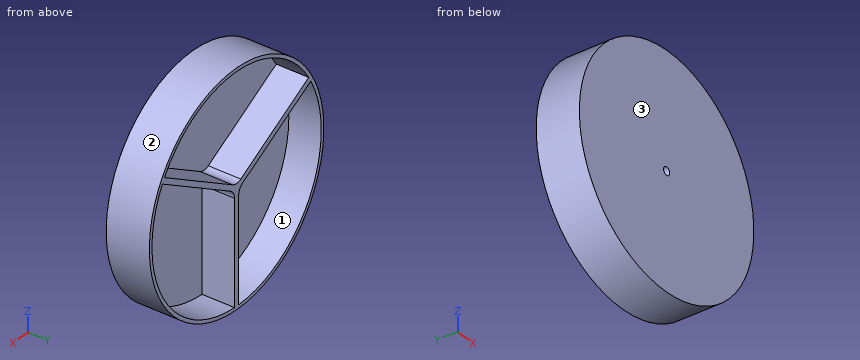
```python
from build123d import *

# Parameters (mm, degrees)
BOSS_EXTRUDE2_DEPTH   = 8
BOSS_EXTRUDE2_2_DEPTH = 8
BOSS_EXTRUDE2_3_DEPTH = 8
SKETCH2_4_R           = 84
BOSS_EXTRUDE3_DEPTH   = 32
SKETCH4_R             = 2.95
CUT_EXTRUDE2_DEPTH    = 8


with BuildPart() as part:
    # Sketch2 → Boss-Extrude2 (new body)
    with BuildSketch(Plane(origin=(0, 0, 0), x_dir=(1, 0, 0), z_dir=(0, 1, 0))):
        with BuildLine():
            Line((-2, 5.579606434), (-2, 81.475456427))
            ThreePointArc((-2, 81.475456427), (-70.623024312, 40.677247166), (-71.479275287, -39.15307401))
            Line((-71.479275287, -39.15307401), (-6, -1.348596796))
            ThreePointArc((-6, -1.348596796), (-3.07179677, 1.579606434), (-2, 5.579606434))
        make_face()
    extrude(amount=BOSS_EXTRUDE2_DEPTH)



with BuildPart() as body_2:
    # Sketch2 → Boss-Extrude2 2 (new body)
    with BuildSketch(Plane(origin=(0, 0, 0), x_dir=(1, 0, 0), z_dir=(0, 1, 0))):
        with BuildLine():
            ThreePointArc((81.5, 0), (58.332023795, 56.917703748), (2, 81.475456427))
            Line((2, 81.475456427), (2, 5.579606434))
            ThreePointArc((2, 5.579606434), (3.07179677, 1.579606434), (6, -1.348596796))
            Line((6, -1.348596796), (71.479275287, -39.15307401))
            ThreePointArc((71.479275287, -39.15307401), (78.95508513, -20.207536516), (81.5, 0))
        make_face()
    extrude(amount=BOSS_EXTRUDE2_2_DEPTH)


with BuildPart() as body_3:
    # Sketch2 → Boss-Extrude2 3 (new body)
    with BuildSketch(Plane(origin=(0, 0, 0), x_dir=(1, 0, 0), z_dir=(0, 1, 0))):
        with BuildLine():
            Line((-4, -4.812698411), (-69.472135836, -42.613053661))
            ThreePointArc((-69.472135836, -42.613053661), (0, -81.5), (69.472135836, -42.613053661))
            Line((69.472135836, -42.613053661), (4, -4.812698411))
            ThreePointArc((4, -4.812698411), (0, -3.740901642), (-4, -4.812698411))
        make_face()
    extrude(amount=BOSS_EXTRUDE2_3_DEPTH)


with BuildPart() as part_1:
    add(part.part)

    add(body_2.part)  # Boss-Extrude3 merges body 2

    add(body_3.part)  # Boss-Extrude3 merges body 3
    # Sketch2_4 → Boss-Extrude3 (add)
    with BuildSketch(Plane(origin=(0, 0, 0), x_dir=(1, 0, 0), z_dir=(0, 1, 0))):
        with Locations(Location((0, 0, 0), (0, 0, 270))):
            Circle(SKETCH2_4_R)
        with BuildLine():
            Line((2, 5.579606434), (2, 81.475456427))
            ThreePointArc((2, 81.475456427), (70.623024312, 40.677247166), (71.479275287, -39.15307401))
            Line((71.479275287, -39.15307401), (6, -1.348596796))
            ThreePointArc((6, -1.348596796), (3.07179677, 1.579606434), (2, 5.579606434))
        make_face(mode=Mode.SUBTRACT)
        with BuildLine():
            Line((4, -4.812698411), (69.472135836, -42.613053661))
            ThreePointArc((69.472135836, -42.613053661), (0, -81.5), (-69.472135836, -42.613053661))
            Line((-69.472135836, -42.613053661), (-4, -4.812698411))
            ThreePointArc((-4, -4.812698411), (0, -3.740901642), (4, -4.812698411))
        make_face(mode=Mode.SUBTRACT)
        with BuildLine():
            Line((-6, -1.348596796), (-71.479275287, -39.15307401))
            ThreePointArc((-71.479275287, -39.15307401), (-70.623024312, 40.677247166), (-2, 81.475456427))
            Line((-2, 81.475456427), (-2, 5.579606434))
            ThreePointArc((-2, 5.579606434), (-3.07179677, 1.579606434), (-6, -1.348596796))
        make_face(mode=Mode.SUBTRACT)
    extrude(amount=BOSS_EXTRUDE3_DEPTH)

    # Sketch4 → Cut-Extrude2 (cut)
    with BuildSketch(Plane(origin=(0, 0, 0), x_dir=(1, 0, 0), z_dir=(0, 1, 0))):
        with Locations(Location((0, 0, 0), (0, 0, 270))):
            Circle(SKETCH4_R)
    extrude(amount=CUT_EXTRUDE2_DEPTH, mode=Mode.SUBTRACT)


solid = part_1.part
```
Geometry: final body of the model. Coordinates: model frame, mm. Face numbers are marked on the shaded views. Coordinates: 2 decimals unless noted, no trailing zeros. Order: outer loops, then holes, each group sorted by start corner. A loop starts at its lowest first (then second) coordinate and runs counter-clockwise, first axis right, second up. Notation, with made-up numbers: (-23, -3) - (-8, -3) arc R24 ccw to (-8, 24) - close; hole circle Ø1 at (-30, 16.25). An arc over 180 degrees is marked (long way). Write each question's results on one line, items separated by ' | '.
(1) First-contact query: pin 1 Ø1 at (x, z) = (-37, -13) entering from +Y; pin 2 Ø3 at (x, z) = (-1, -1) entering from -Y; pin 3 Ø4 at (x, y) = (-27.5, 7) entering from -Z. Flat tips, straight axial feed; report the tip coordinate or a pass-through.
Values found:
pin 1: stops at y = 8 | pin 2: stops at y = 8 | pin 3: stops at z = -80.04
(2) Line query: line 1 (X direction, y = 5, z = 0); line 2 (X direction, y = 25, z = -51.5); line 3 (X direction, y = 25, z = -24.5). Output: solid intervals per line, ascending. Write a range as [from, to].
Values found:
line 1: x = [-84, -2.95], [2.95, 84] | line 2: x = [-66.36, -63.17], [-2, 2], [63.17, 66.36] | line 3: x = [-80.35, -77.73], [-2, 2], [77.73, 80.35]
(3) Mould query, pull axis Z, two halves, no side actions, for the marked faces 1, 2 and 3. Classes: +Z half, -Z half, draft (parallel to the pull), parting line (faces both ways), or undercut.
Values found:
face 1: undercut | face 2: parting line | face 3: draft
(4) Section query D-D, the plane z = 19. Return the cut outline in (x, y), plus the area to 3 significant figures.
Values found:
outline: (-81.82, 0) - (81.82, 0) - (81.82, 32) - (79.25, 32) - (79.25, 8) - (36.57, 8) - (36.57, 32) - (28.57, 32) - (28.57, 8) - (-28.57, 8) - (-28.57, 32) - (-36.57, 32) - (-36.57, 8) - (-79.25, 8) - (-79.25, 32) - (-81.82, 32) - close | area: 1,820 mm²
(5) Section query C-C, the plane y = 5. Return the cut outline in (x, z), plus the area to 3 significant figures.
Values found:
outline: circle Ø168 at (0, 0); hole circle Ø5.9 at (0, 0) | area: 22,100 mm²
(6) Section query B-B, the plane x = 0. Return the cut outline in (y, z), plus the area to 3 significant figures.
Values found:
outline: (0, -84) - (32, -84) - (32, 3.74) - (8, 3.74) - (8, 81.5) - (32, 81.5) - (32, 84) - (0, 84) - (0, 2.95) - (8, 2.95) - (8, -2.95) - (0, -2.95) - close | area: 3,460 mm²
(7) Section query A-A, the plane y = 21. Return the cut outline in (x, z).
Values found:
outline: circle Ø168 at (0, 0); hole (-71.48, 39.15) arc R81.5 ccw to (-2, -81.48) - (-2, -5.58) arc R8 ccw to (-6, 1.35) - close; hole (-69.47, 42.61) - (-4, 4.81) arc R8 ccw to (4, 4.81) - (69.47, 42.61) arc R81.5 ccw to start; hole (2, -81.48) arc R81.5 ccw to (71.48, 39.15) - (6, 1.35) arc R8 ccw to (2, -5.58) - close
